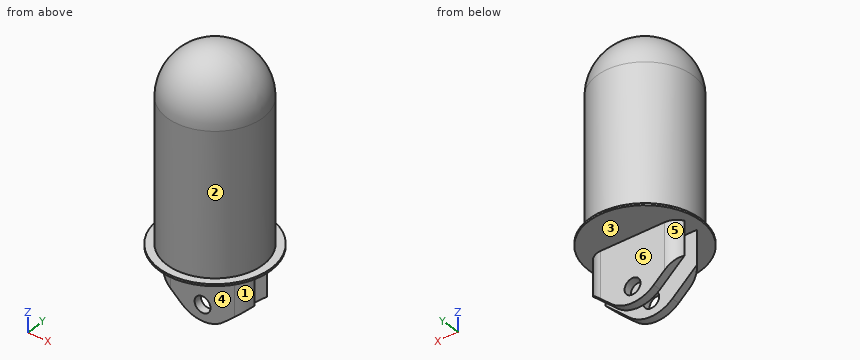
```python
from build123d import *

# Parameters (mm, degrees)
F0_R        = 38.1
F1_DEPTH    = 152.4
F2_R        = 38.1
F4_DEPTH    = 12.7
F5_T1_DEPTH = 57.15
F6_W        = 12.7
F6_H        = 50.8
F7_DEPTH    = 38.1
F0_R_2      = 44.45
F8_DEPTH    = 1.5875


# Not quite as in the source:
# - a fillet or chamfer that OpenCascade refuses, or shapes differently, is made with other operations: its cross-section is extruded or revolved along the edge and cut away or added


with BuildPart() as f1:
    # F0 (on Top) → F1 (new body)
    with BuildSketch(Plane.XY):
        Circle(F0_R)
    extrude(amount=F1_DEPTH)

    # F2
    f2_edges = [f1.edges().sort_by_distance(p)[0] for p in [
        (-38.1, 0, 152.4),
    ]]
    fillet(f2_edges, radius=F2_R)

    # F3 (on Front) → F4 (join, symmetric)
    with BuildSketch(Plane.XZ):
        with BuildLine():
            Line((16.9333333333, -44.3320422095), (38.1, -25.4))
            Line((38.1, -25.4), (38.1, 0))
            Line((38.1, 0), (0, 0))
            Line((0, 0), (-38.1, 0))
            Line((-38.1, 0), (-38.1, -25.4))
            Line((-38.1, -25.4), (-16.9333333333, -44.3320422095))
            ThreePointArc((-16.9333333333, -44.3320422095), (0, -50.8), (16.9333333333, -44.3320422095))
        make_face()
        with BuildLine():
            ThreePointArc((6.35, -38.1), (-4.4901280605, -42.5901280605), (0, -31.75))
            ThreePointArc((0, -31.75), (4.4901280605, -33.6098719395), (6.35, -38.1))
        make_face(mode=Mode.SUBTRACT)
    extrude(amount=F4_DEPTH, both=True)

    # F5: fillet of radius 12.7 on 4 edges, made by hand

    # F5_s2 → F5_t1 (cut)
    with BuildSketch(Plane.XY.offset(-57.15)):
        with BuildLine():
            ThreePointArc((38.1, 0), (34.3802561211, -8.9802561211), (25.4, -12.7))
            Line((25.4, -12.7), (38.1, -12.7))
            Line((38.1, -12.7), (38.1, 0))
        make_face()
        with BuildLine():
            ThreePointArc((38.1, 0), (34.3802561211, 8.9802561211), (25.4, 12.7))
            Line((25.4, 12.7), (38.1, 12.7))
            Line((38.1, 12.7), (38.1, 0))
        make_face()
        with BuildLine():
            ThreePointArc((-25.4, 12.7), (-34.3802561211, 8.9802561211), (-38.1, 0))
            Line((-38.1, 0), (-38.1, 12.7))
            Line((-38.1, 12.7), (-25.4, 12.7))
        make_face()
        with BuildLine():
            ThreePointArc((-38.1, 0), (-34.3802561211, -8.9802561211), (-25.4, -12.7))
            Line((-25.4, -12.7), (-38.1, -12.7))
            Line((-38.1, -12.7), (-38.1, 0))
        make_face()
    extrude(amount=F5_T1_DEPTH, mode=Mode.SUBTRACT)

    # F6 (on Right) → F7 (cut, symmetric)
    with BuildSketch(Plane.YZ):
        with Locations((0, -25.4)):
            Rectangle(F6_W, F6_H)
    extrude(amount=F7_DEPTH, both=True, mode=Mode.SUBTRACT)

    # F0 (on Top) → F8 (join)
    with BuildSketch(Plane.XY):
        Circle(F0_R_2)
        Circle(F0_R, mode=Mode.SUBTRACT)
    extrude(amount=F8_DEPTH)


solid = f1.part
```
Work out the finished part from the listing and answer in its coordinate system (mm). Face numbers are marked on the shaded views. A direction names the side the tool comes from. Give positions to 0.01 mm unless a question says otherwise; leave off trailing zeros. Loops run counter-clockwise (first coordinate to the right, second up) from the corner with the lowest first, then second, coordinate; pieces in that order, holes last. Notation, with made-up numbers: (16.25, -38) - (32.25, -38) arc R15 cw to (32.25, -29) - close; hole circle Ø10 at (-20, 80). An arc over 180 degrees is marked (long way). One line per question, with ' | ' between items.
(1) A tool of negligible diameter and unlimited length cuts with its end or side. For the marked faces 4, 5 and 6, from which of +Z, -Z, +X, -X, +Y, -Y can it reach the whole face along a straight path? Write none if from no direction.
Recorded:
face 4: -Z, +X, -X, -Y | face 5: -Z, -X, +Y | face 6: -Z, +X, -X, +Y
(2) The part is cut by section D-D (z = 89). Write down the section's boundary in (x, y), then the cut area to 3 significant figures.
Recorded:
outline: circle Ø76.2 at (0, 0) | area: 4,560 mm²
(3) The part is cut by section C-C (y = 0). Write down the section's boundary in (x, z), then the cut area to 3 significant figures.
Recorded:
outline: (-44.45, 0) - (44.45, 0) - (44.45, 1.59) - (38.1, 1.59) - (38.1, 114.3) arc R38.1 ccw to (-38.1, 114.3) - (-38.1, 1.59) - (-44.45, 1.59) - close | area: 11,000 mm²
(4) The part is cut by section B-B (x = 0). Write down the section's boundary in (y, z), then the cut area to 3 significant figures.
Recorded:
outline: (-44.45, 0) - (-12.7, 0) - (-12.7, -31.75) - (-6.35, -31.75) - (-6.35, 0) - (6.35, 0) - (6.35, -31.75) - (12.7, -31.75) - (12.7, 0) - (44.45, 0) - (44.45, 1.59) - (38.1, 1.59) - (38.1, 114.3) arc R38.1 ccw to (-38.1, 114.3) - (-38.1, 1.59) - (-44.45, 1.59) - close; (-12.7, -50.8) - (-6.35, -50.8) - (-6.35, -44.45) - (-12.7, -44.45) - close; (6.35, -50.8) - (12.7, -50.8) - (12.7, -44.45) - (6.35, -44.45) - close | area: 11,500 mm²
(5) The mould has two halves that part along Y. Classify the marked faces 1, 2 and 3: +Y half, -Y half, draft (parallel to the pull), parting line (faces both ways), or undercut.
Recorded:
face 1: -Y half | face 2: parting line | face 3: undercut
(6) Each of these flat-tipped pins is pushed along its axis until it touches: pin 1 Ø12 at (x, y) = (20, 9.5) entering from +Z; pin 2 Ø8 at (x, y) = (3.5, 8.5) entering from -Z; pin 3 Ø15 at (x, z) = (4.5, -36) entering from +Y. Where does it stop, or does it pass through?
Recorded:
pin 1: stops at z = 148.81 | pin 2: stops at z = -50.8 | pin 3: stops at y = 12.7
(7) The part is cut by section A-A (z = -4). Write down the section's boundary in (x, y).
Recorded:
outline: (-36.4, -6.35) arc R12.7 ccw to (-25.4, -12.7) - (25.4, -12.7) arc R12.7 ccw to (36.4, -6.35) - close; (-36.4, 6.35) - (36.4, 6.35) arc R12.7 ccw to (25.4, 12.7) - (-25.4, 12.7) arc R12.7 ccw to start
(8) Straight lines are drawn through the part: probe 1 along Y at (x, z) = (-1, -10.5); probe 2 along Z at (x, y) = (0, 7); probe 3 along Z at (x, y) = (-21, 37). For each, find the intervals that lie inside material, in ascending order.
Recorded:
probe 1: y = -12.7 to -6.35, 6.35 to 12.7 | probe 2: z = -50.8 to -44.45, -31.75 to 151.75 | probe 3: z = 0 to 1.59
